Part print with two shaded views. Sizes in mm from the minimum x, y, z corner. A direction names the side the tool comes from. Coordinates: 2 decimals unless noted, no trailing zeros. Loops run counter-clockwise (first coordinate to the right, second up) from the corner with the lowest first, then second, coordinate; pieces in that order, holes last. Notation, with made-up numbers: (-6, 47.5) -> (18, 47.5) arc R14 ccw to (18, 63.5) -> close; hole circle Ø6 at (-6.75, 47.5). An arc over 180 degrees is marked (long way). Write each question's results on one line, items separated by ' | '.
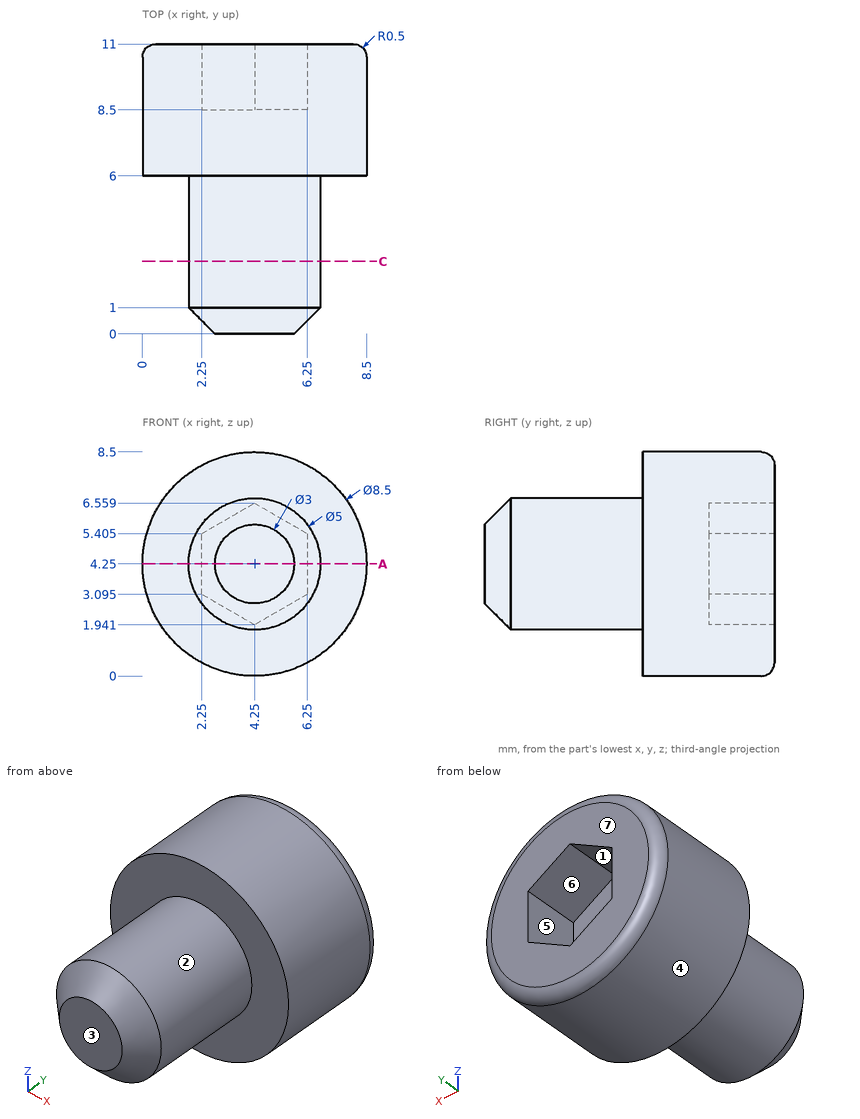
Q1. Which spindle directions (+Z, -Z, +X, -X, +Y, -Y) get a long thin tool onto all of the face, cutting with end or side? Do the marked faces 1, 2 and 3. Say none if no direction does.
Results are:
face 1: +Y | face 2: -Y | face 3: +Z, -Z, +X, -X, -Y
Q2. Cut at C-C on y = 2.75. Write the cut outline in (x, z), and give its area (3 significant figures).
Results are:
outline: circle Ø5 at (4.25, 4.25) | area: 19.6 mm^2
Q3. Cut at A-A on z = 4.25. Write the cut outline in (x, y), and give its area (3 significant figures).
Results are:
outline: (0, 6) -> (1.75, 6) -> (1.75, 1) -> (2.75, 0) -> (5.75, 0) -> (6.75, 1) -> (6.75, 6) -> (8.5, 6) -> (8.5, 10.5) arc R0.5 ccw to (8, 11) -> (6.25, 11) -> (6.25, 8.5) -> (2.25, 8.5) -> (2.25, 11) -> (0.5, 11) arc R0.5 ccw to (0, 10.5) -> close | area: 61.4 mm^2
Q4. Drop flat-ended pins along their axis: pin 1 (3 mm diameter, centred on y = 3, z = 5, fed in from -X); pin 2 (1 mm diameter, centred on y = 10, z = 1, fed in from -X); pin 3 (1 mm diameter, centred on y = 9, z = 5.5, fed in from +X). Give the stop position or say it passes through.
Results are:
pin 1: x = 1.75 | pin 2: x = 1.01 | pin 3: x = 8.43
Q5. Pull direction Z, two halves, no side cores. Call the marked faces 4, 5, 6 and 7: +Z half, -Z half, draft (parallel to the pull), parting line (faces both ways), or undercut.
Results are:
face 4: parting line | face 5: undercut | face 6: undercut | face 7: draft
Q6. Wall check: L1, parallel to Y at x = 3, z = 7.5; L2, parallel to X at y = 10.5, z = 4.75; L3, parallel to X at y = 9.5, z = 5. Give the ranges that are in metal, low to high. Write a range as from..to.
Results are:
L1: 6..11 | L2: 0.03..2.25, 6.25..8.47 | L3: 0.07..2.25, 6.25..8.43
